The model under review builds one solid part; all positions refer to its coordinate system, in mm. Face numbers are marked on the shaded views. Coordinates: 2 decimals unless noted, no trailing zeros. Loops run counter-clockwise (first coordinate to the right, second up) from the corner with the lowest first, then second, coordinate; pieces in that order, holes last. Notation, with made-up numbers: (-12, 11.25) - (11, 11.25) arc R25 cw to (11, 31.25) - close; hole circle Ø5 at (49.5, 66.5). An arc over 180 degrees is marked (long way). Answer in a Markdown table with one row per item. Add a question column.
(1) Mouldability with a two-part tool opening along Y and no side actions: class the marked faces 1 and 2 as +Y half, -Y half, draft (parallel to the pull), parting line (faces both ways), or undercut.
(2) We need section B-B on x = -18.5. Write out the cut boundary in (y, z).
(3) For P1, Ø10, axis at x = -18.5, z = -16.5, coming from the +Y side; P2, Ø1.5, axis at x = -8.5, y = 6, coming from the -Z side; P3, Ø6, axis at x = 29, y = 5.5, coming from the -Z side, all flat-tipped, find the tip position at first contact; note any pin that passes through.
(4) We need section A-A on x = 32.5. Write out the cut boundary in (y, z).
(5) For line 1 along Y through (x, z) = (-44, -10); line 2 along Z through (x, y) = (-5.5, 14); line 3 along Y through (x, z) = (30, 14.5), list the stretches that pass through material, from the lowest coordinate up.
from build123d import *

# Parameters (mm, degrees)
F3_SIZE = 0.508


with BuildPart() as f1:
    # F0 (on Front) → F1 (revolve)
    with BuildSketch(Plane.XZ):
        Polygon((50.8, 25.4), (0, 25.4), (0, 22.098), (50.8, 22.86), align=None)
    revolve(axis=Axis((-51.9470935156, 0, 0), (-1, 0, 0)))

    # F2: F1 across face


with BuildPart() as f1_1:
    add(f1.part)
    add(f1.part.mirror(Plane(origin=(0, 0, 0), x_dir=(0, -1, 0), z_dir=(-1, 0, 0))))

    # F3
    f3_edges = [f1_1.edges().sort_by_distance(p)[0] for p in [
        (-50.8, 0, -22.86),
        (50.8, 0, -22.86),
    ]]
    chamfer(f3_edges, length=F3_SIZE)


solid = f1_1.part
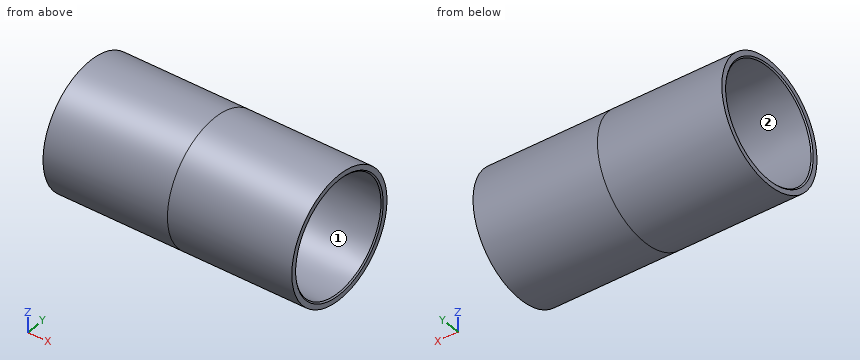
Outcome:
| question | item | result |
|---|---|---|
| 1 | face 1 | undercut |
| 1 | face 2 | undercut |
| 2 | outline | circle Ø50.8 at (0, 0); hole circle Ø44.75 at (0, 0) |
| 3 | P1 | y = 22.65 |
| 3 | P2 | z = -24.85 |
| 3 | P3 | z = -25.28 |
| 4 | outline | circle Ø50.8 at (0, 0); hole circle Ø45.17 at (0, 0) |
| 5 | line 1 | -23.35 to -20.44, 20.44 to 23.35 |
| 5 | line 2 | -21.19 to -17.2, 17.2 to 21.19 |
| 5 | line 3 | -20.85 to -17.27, 17.27 to 20.85 |
